from build123d import *

# Parameters (mm, degrees)
BOSS_EXTRUDE1_DEPTH = 150
SKETCH2_R           = 2.5
BOSS_EXTRUDE2_DEPTH = 25
CUT_EXTRUDE1_START  = -7
SKETCH3_R           = 2.5
SKETCH3_R_2         = 1.733910687
CUT_EXTRUDE1_DEPTH  = 7


with BuildPart() as part:
    # Sketch1 → Boss-Extrude1 (new body)
    with BuildSketch(Plane(origin=(0, 0, 0), x_dir=(0, 0, -1), z_dir=(1, 0, 0))):
        Polygon((-50, 35), (50, 35), (50, -15), (20, -15), (20, 0), (-20, 0), (-20, -15), (-50, -15), align=None)
    extrude(amount=-BOSS_EXTRUDE1_DEPTH)

    # Sketch2 → Boss-Extrude2 (add)
    with BuildSketch(Plane.XY.offset(50)):
        with Locations((-75, 10)):
            Circle(SKETCH2_R)
    extrude(amount=BOSS_EXTRUDE2_DEPTH)

    # Sketch3 → Cut-Extrude1 (cut)
    with BuildSketch(Plane.XY.offset(75).offset(CUT_EXTRUDE1_START)):
        with Locations((-75, 10)):
            Circle(SKETCH3_R)
        with Locations((-75, 10)):
            Circle(SKETCH3_R_2, mode=Mode.SUBTRACT)
    extrude(amount=-CUT_EXTRUDE1_DEPTH, mode=Mode.SUBTRACT)


solid = part.part
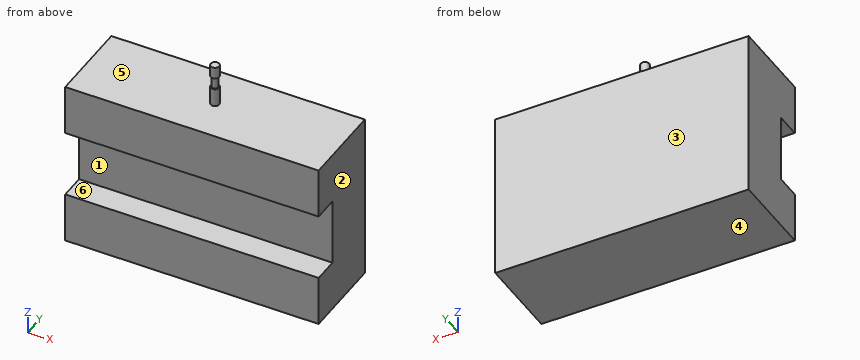
Could you check a few things on this model? Use its own coordinates, in mm. Face numbers are marked on the shaded views. A direction names the side the tool comes from. Round coordinates to 2 decimals unless told otherwise and drop trailing zeros. Order: outer loops, then holes, each group sorted by start corner. A loop starts at its lowest first (then second) coordinate and runs counter-clockwise, first axis right, second up.
(1) Imagine slicing it at A-A (y = -5). Write out the boundary of the cut face in (x, z), plus the area to 3 significant figures.
Response values:
outline: (-150, -50) - (0, -50) - (0, -20) - (-150, -20) - close; (-150, 20) - (0, 20) - (0, 50) - (-150, 50) - close
area: 9,000 mm2
(2) Imagine slicing it at B-B (x = -17). Write out the boundary of the cut face in (y, z).
Response values:
outline: (-15, -50) - (35, -50) - (35, 50) - (-15, 50) - (-15, 20) - (0, 20) - (0, -20) - (-15, -20) - close
(3) Which directions (+Z, -Z, +X, -X, +Y, -Y) give clear straight access to the entire face, cutting with the end or side of a thin tool? Please do the marked faces 1 and 2.
Response values:
face 1: +X, -X, -Y
face 2: +Z, -Z, +X, +Y, -Y
(4) Imagine slicing it at C-C (y = 10). Write out the boundary of the cut face in (x, z).
Response values:
outline: (-150, -50) - (0, -50) - (0, 50) - (-72.5, 50) - (-72.5, 61) - (-73.27, 61) - (-73.27, 68) - (-72.5, 68) - (-72.5, 75) - (-77.5, 75) - (-77.5, 68) - (-76.73, 68) - (-76.73, 61) - (-77.5, 61) - (-77.5, 50) - (-150, 50) - close
(5) If we mould it in two halves opening along Z, with no side actions, what happens to the marked faces 3, 4, 5 and 6? For each: released by +Z, released by -Z, zero draft, split by the parting line, or undercut.
Response values:
face 3: zero draft
face 4: released by -Z
face 5: released by +Z
face 6: undercut
(6) Please list where these lines run through material, in increasing order: line 1 along Z through (x, y) = (-48.5, 20.5); line 2 along Z through (x, y) = (-25.5, -2); line 3 along Y through (x, z) = (-97.5, -19.5).
Response values:
line 1: z = -50 to 50
line 2: z = -50 to -20, 20 to 50
line 3: y = 0 to 35
(7) Imagine slicing it at D-D (x = -75). Write out the boundary of the cut face in (y, z).
Response values:
outline: (-15, -50) - (35, -50) - (35, 50) - (12.5, 50) - (12.5, 61) - (11.73, 61) - (11.73, 68) - (12.5, 68) - (12.5, 75) - (7.5, 75) - (7.5, 68) - (8.27, 68) - (8.27, 61) - (7.5, 61) - (7.5, 50) - (-15, 50) - (-15, 20) - (0, 20) - (0, -20) - (-15, -20) - close
(8) I'm going to push flat-ended pins straight in: pin 1 (12 mm diameter, centred on x = -84, z = -7.5, fed in from -Y); pin 2 (4.5 mm diameter, centred on x = -112, y = -8.5, fed in from +Z). Where does each tip first touch, or does it pass through?
Response values:
pin 1: stops at y = 0
pin 2: stops at z = 50
